```python
from build123d import *

# Parameters (mm, degrees)
SKETCH2_R           = 34.410626859
SKETCH2_R_2         = 16.637
BOSS_EXTRUDE1_DEPTH = 101.6
SKETCH3_W           = 16.158329911
SKETCH3_H           = 33.912544257
BOSS_EXTRUDE2_DEPTH = 25.4
SKETCH4_R           = 4.896317789
BOSS_EXTRUDE3_DEPTH = 50.8
BOSS_EXTRUDE3_TAPER = -8
FILLET1_R           = 7.62


with BuildPart() as part:
    # Sketch2 → Boss-Extrude1 (new body)
    with BuildSketch(Plane.XY):
        Circle(SKETCH2_R)
        Circle(SKETCH2_R_2, mode=Mode.SUBTRACT)
    extrude(amount=BOSS_EXTRUDE1_DEPTH)

    # Sketch3 → Boss-Extrude2 (add)
    with BuildSketch(Plane.XY.offset(101.6)):
        with Locations((29.723347614, 0.099742777)):
            Rectangle(SKETCH3_W, SKETCH3_H)
    extrude(amount=-BOSS_EXTRUDE2_DEPTH)

    # Sketch4 → Boss-Extrude3 (add)
    with BuildSketch(Plane(origin=(37.802512569, 0, 0), x_dir=(0, 0, -1), z_dir=(1, 0, 0))):
        with Locations((-87.324916431, 1.22659491)):
            Circle(SKETCH4_R)
    extrude(amount=BOSS_EXTRUDE3_DEPTH, taper=BOSS_EXTRUDE3_TAPER)

    # Fillet1
    fillet1_edges = [part.edges().sort_by_distance(p)[0] for p in [
        (88.602512569, 1.22659491, 99.360708623),
    ]]
    fillet(fillet1_edges, radius=FILLET1_R)


solid = part.part
```
Model file for the job. Use its own axes, mm. A direction names the side the tool comes from. Coordinates: 2 decimals unless noted, no trailing zeros. Loops run counter-clockwise (first coordinate to the right, second up) from the corner with the lowest first, then second, coordinate; pieces in that order, holes last. Notation, with made-up numbers: M -5.75,-20.5 L 9.25,-20.5 A27 cw 9.25,8.5 Z; hole C 38,74.25 d10. An arc over 180 degrees is marked long. Use CSV: the item, a comma, the result in double quotes. Start each with the question number.
1. Tool access for faces 4 (the flat face through (34, -16.857, 89)), 5 (the conical face through (59.16, 6.56, 93.15)), 6 (the flat face through (36, 0, 76.2)), 7 (the flat face through (34, 17.056, 89)): list every direction of +Z, -Z, +X, -X, +Y, -Y with a clear straight run to the whole face (end or side of a thin tool).
2. Flat gauge pins, fed straight in: pin 1 (4 mm diameter, centred on x = 35.5, z = 90, fed in from +Y); pin 2 (1 mm diameter, centred on y = 11, z = 17.5, fed in from +X); pin 3 (1.5 mm diameter, centred on y = -26, z = 69, fed in from -X). Where does each tip first touch, or does it go through?
3. Two-plate mould, pull along X, no slides. Class faces 1 (the cylindrical face through (-34.377, 1.513, 50.089)), 2 (the cylindrical face through (-2.166, 16.495, 50.089)), 3 (the flat face through (15, 8, 0)): pulls with the +X half, pulls with the -X half, needs draft (parallel to the pull), parting line crosses it, or undercut.
4. Band-saw the part on A-A, the plane x = 0. List the corners of the cut face in (y, z), then the cut area to 3 significant figures.
5. Band-saw the part on D-D, the plane x = -12.5. List the corners of the cut face in (y, z).
6. Probe probe 1 along Y at (x, z) = (0, 47); probe 2 along X at (y, z) = (-13.5, 64); probe 3 along X at (y, z) = (10, 73). List the from-to ranges inside material, lowest first. Write a range as [from, to].
7. Band-saw the part on C-C, the plane z = 32. List the corners of the cut face in (x, y), then the cut area to 3 significant figures.
8. Band-saw the part on B-B, the plane y = 14. List the corners of the cut face in (x, z).
Entries:
1,face 4,"+Z, -Z, +X, -Y"
1,face 5,"none"
1,face 6,"-Z, +X"
1,face 7,"+Z, -Z, +X, +Y"
2,pin 1,"stops at y = 17.06"
2,pin 2,"stops at x = 32.77"
2,pin 3,"stops at x = -23.38"
3,face 1,"parting line crosses it"
3,face 2,"undercut"
3,face 3,"needs draft"
4,outline,"M -34.41,0 L -16.64,0 L -16.64,101.6 L -34.41,101.6 Z; M 16.64,0 L 34.41,0 L 34.41,101.6 L 16.64,101.6 Z"
4,area,"3,610 mm2"
5,outline,"M -32.06,0 L -10.98,0 L -10.98,101.6 L -32.06,101.6 Z; M 10.98,0 L 32.06,0 L 32.06,101.6 L 10.98,101.6 Z"
6,probe 1,"y = [-34.41, -16.64], [16.64, 34.41]"
6,probe 2,"x = [-31.65, -9.72], [9.72, 31.65]"
6,probe 3,"x = [-32.93, -13.3], [13.3, 32.93]"
7,outline,"C 0,0 d68.82; hole C 0,0 d33.27"
7,area,"2,850 mm2"
8,outline,"M -31.43,0 L -8.99,0 L -8.99,101.6 L -31.43,101.6 Z; M 8.99,0 L 31.43,0 L 31.43,76.2 L 37.8,76.2 L 37.8,101.6 L 8.99,101.6 Z"
